from build123d import *

# Parameters (mm, degrees)
SKETCH2_R           = 1.75
SKETCH2_R_2         = 1.995
BOSS_EXTRUDE1_DEPTH = 4
SKETCH4_R           = 1.3
SKETCH4_R_2         = 2.4
CUT_EXTRUDE1_DEPTH  = 5


with BuildPart() as part:
    # Sketch2 → Boss-Extrude1 (new body)
    with BuildSketch(Plane.XY):
        with BuildLine():
            ThreePointArc((30.75, -4), (34.75, 0), (30.75, 4))
            Line((30.75, 4), (14.072558403, 4))
            ThreePointArc((14.072558403, 4), (14.06038767, 4.04257326), (14.048088143, 4.085109489))
            ThreePointArc((14.048088143, 4.085109489), (12.709169027, 4.272836063), (11.365584201, 4.122086336))
            ThreePointArc((11.365584201, 4.122086336), (11.169703548, 4.626642697), (10.951436862, 5.12192646))
            ThreePointArc((10.951436862, 5.12192646), (12.008090957, 5.965388247), (12.82210701, 7.044889767))
            ThreePointArc((12.82210701, 7.044889767), (12.669951657, 7.315), (12.51210701, 7.581825517))
            ThreePointArc((12.51210701, 7.581825517), (11.170223244, 7.416617696), (9.911436862, 6.9232593))
            ThreePointArc((9.911436862, 6.9232593), (9.591641884, 7.359925677), (9.252623584, 7.781841479))
            ThreePointArc((9.252623584, 7.781841479), (10.05496909, 8.870045207), (10.561852666, 10.123446462))
            ThreePointArc((10.561852666, 10.123446462), (10.344972209, 10.344972209), (10.123446462, 10.561852666))
            ThreePointArc((10.123446462, 10.561852666), (8.870045207, 10.05496909), (7.781841479, 9.252623584))
            ThreePointArc((7.781841479, 9.252623584), (7.359925677, 9.591641884), (6.9232593, 9.911436862))
            ThreePointArc((6.9232593, 9.911436862), (7.416617696, 11.170223244), (7.581825517, 12.51210701))
            ThreePointArc((7.581825517, 12.51210701), (7.315, 12.669951657), (7.044889767, 12.82210701))
            ThreePointArc((7.044889767, 12.82210701), (5.965388247, 12.008090957), (5.12192646, 10.951436862))
            ThreePointArc((5.12192646, 10.951436862), (4.626642697, 11.169703548), (4.122086336, 11.365584201))
            ThreePointArc((4.122086336, 11.365584201), (4.272836063, 12.709169027), (4.085109489, 14.048088143))
            ThreePointArc((4.085109489, 14.048088143), (3.78652263, 14.131494839), (3.486235477, 14.208555951))
            ThreePointArc((3.486235477, 14.208555951), (2.654199937, 13.14288127), (2.112960617, 11.903927815))
            ThreePointArc((2.112960617, 11.903927815), (1.578061664, 11.986568374), (1.04, 12.04518576))
            ThreePointArc((1.04, 12.04518576), (0.837867713, 13.382005944), (0.31, 14.626715284))
            ThreePointArc((0.31, 14.626715284), (0, 14.63), (-0.31, 14.626715284))
            ThreePointArc((-0.31, 14.626715284), (-0.837867713, 13.382005944), (-1.04, 12.04518576))
            ThreePointArc((-1.04, 12.04518576), (-1.578061664, 11.986568374), (-2.112960617, 11.903927815))
            ThreePointArc((-2.112960617, 11.903927815), (-2.654199937, 13.14288127), (-3.486235477, 14.208555951))
            ThreePointArc((-3.486235477, 14.208555951), (-3.78652263, 14.131494839), (-4.085109489, 14.048088143))
            ThreePointArc((-4.085109489, 14.048088143), (-4.272836063, 12.709169027), (-4.122086336, 11.365584201))
            ThreePointArc((-4.122086336, 11.365584201), (-4.626642697, 11.169703548), (-5.12192646, 10.951436862))
            ThreePointArc((-5.12192646, 10.951436862), (-5.965388247, 12.008090957), (-7.044889767, 12.82210701))
            ThreePointArc((-7.044889767, 12.82210701), (-7.315, 12.669951657), (-7.581825517, 12.51210701))
            ThreePointArc((-7.581825517, 12.51210701), (-7.416617696, 11.170223244), (-6.9232593, 9.911436862))
            ThreePointArc((-6.9232593, 9.911436862), (-7.359925677, 9.591641884), (-7.781841479, 9.252623584))
            ThreePointArc((-7.781841479, 9.252623584), (-8.870045207, 10.05496909), (-10.123446462, 10.561852666))
            ThreePointArc((-10.123446462, 10.561852666), (-10.344972209, 10.344972209), (-10.561852666, 10.123446462))
            ThreePointArc((-10.561852666, 10.123446462), (-10.05496909, 8.870045207), (-9.252623584, 7.781841479))
            ThreePointArc((-9.252623584, 7.781841479), (-9.591641884, 7.359925677), (-9.911436862, 6.9232593))
            ThreePointArc((-9.911436862, 6.9232593), (-11.170223244, 7.416617696), (-12.51210701, 7.581825517))
            ThreePointArc((-12.51210701, 7.581825517), (-12.669951657, 7.315), (-12.82210701, 7.044889767))
            ThreePointArc((-12.82210701, 7.044889767), (-12.008090957, 5.965388247), (-10.951436862, 5.12192646))
            ThreePointArc((-10.951436862, 5.12192646), (-11.169703548, 4.626642697), (-11.365584201, 4.122086336))
            ThreePointArc((-11.365584201, 4.122086336), (-12.709169027, 4.272836063), (-14.048088143, 4.085109489))
            ThreePointArc((-14.048088143, 4.085109489), (-14.131494839, 3.78652263), (-14.208555951, 3.486235477))
            ThreePointArc((-14.208555951, 3.486235477), (-13.14288127, 2.654199937), (-11.903927815, 2.112960617))
            ThreePointArc((-11.903927815, 2.112960617), (-11.986568374, 1.578061664), (-12.04518576, 1.04))
            ThreePointArc((-12.04518576, 1.04), (-13.382005944, 0.837867713), (-14.626715284, 0.31))
            ThreePointArc((-14.626715284, 0.31), (-14.63, 0), (-14.626715284, -0.31))
            ThreePointArc((-14.626715284, -0.31), (-13.382005944, -0.837867713), (-12.04518576, -1.04))
            ThreePointArc((-12.04518576, -1.04), (-11.986568374, -1.578061664), (-11.903927815, -2.112960617))
            ThreePointArc((-11.903927815, -2.112960617), (-13.14288127, -2.654199937), (-14.208555951, -3.486235477))
            ThreePointArc((-14.208555951, -3.486235477), (-14.131494839, -3.78652263), (-14.048088143, -4.085109489))
            ThreePointArc((-14.048088143, -4.085109489), (-12.709169027, -4.272836063), (-11.365584201, -4.122086336))
            ThreePointArc((-11.365584201, -4.122086336), (0.064808849, -12.089826294), (11.409123542, -4))
            Line((11.409123542, -4), (30.75, -4))
        make_face()
        Circle(SKETCH2_R, mode=Mode.SUBTRACT)
        with Locations((30.75, 0)):
            Circle(SKETCH2_R_2, mode=Mode.SUBTRACT)
    extrude(amount=BOSS_EXTRUDE1_DEPTH)

    # Sketch4 → Cut-Extrude1 (cut, through all)
    with BuildSketch(Plane.XY.offset(4)):
        with Locations((4.5, 0)):
            Circle(SKETCH4_R)
        with Locations((-4.5, 0)):
            Circle(SKETCH4_R)
        Circle(SKETCH4_R_2)
    extrude(amount=-CUT_EXTRUDE1_DEPTH, mode=Mode.SUBTRACT)


solid = part.part
Design review of the part built by this model. Coordinates are the model's own, in mm. A direction names the side the tool comes from. Round coordinates to 2 decimals unless told otherwise and drop trailing zeros. Write each loop counter-clockwise with the first axis right and the second up, starting at its lowest first coordinate (ties: lowest second). Pieces come first, ordered by that corner, then holes. Notation, with made-up numbers: M 46,15 L 71,15 A26 cw 71,51 Z; hole C 6,-28 d4. An arc over 180 degrees is marked long. One line per item, written item: value. Start each with the question number.
1. Take a section at B-B on x = 18.5. State the section outline as (y, z) points.
2. Clearance check with flat-ended pins moving along their axes: P1, Ø5.5, axis at x = 0, y = 0, coming from the -Z side; P2, Ø1.5, axis at x = 7, z = 0.5, coming from the -Y side; P3, Ø2, axis at x = 23, z = 2, coming from the -Y side; P4, Ø1.5, axis at y = 10, z = 2.5, coming from the +X side. State where each tip first meets the part, or that it passes through.
3. To check wall thickness, follow probe 1 along Y at (x, z) = (30.75, 2.2) (3 decimals); probe 2 along X at (y, z) = (-1.5, 1.85); probe 3 along Y at (x, z) = (0, 2.7). State the ranges of each line that lie inside material, in increasing order. Write a range as from..to.
4. Draft analysis for pull direction X (two halves, no side actions). For faces 4 (the face through (-8.853, 10.046, 1.972)), 5 (the face through (-11.986, 1.586, 1.972)), 6 (the face through (10.046, 8.853, 1.972)), state which applies: pulls with the +X half, pulls with the -X half, needs draft (parallel to the pull), parting line crosses it, or undercut.
5. For faces 1 (the face through (-10.064, 8.887, 1.972)), 2 (the face through (-12.69, 4.273, 1.972)), 3 (the face through (2.664, 13.159, 1.972)), list the 3-axis set-ups (+Z, -Z, +X, -X, +Y, -Y) from which the entire face can be reached by the end or side of a thin tool; tool diameter is ignored.
6. Take a section at A-A on z = 1.5. State how many separate pieces and enclosed holes the cut face has, then the cut area to 3 significant figures.
7. Take a section at C-C on y = -6.75. State the section outline as (x, z) points.
Computed:
1. outline: M -4,0 L 4,0 L 4,4 L -4,4 Z
2. P1: stops at z = 0
2. P2: stops at y = -10.35
2. P3: stops at y = -4
2. P4: stops at x = 10.56
3. probe 1: y = -4..-1.995, 1.995..4
3. probe 2: x = -12..-1.87, 1.87..29.43, 32.07..34.46
3. probe 3: y = -12.09..-2.4, 2.4..14.63
4. face 4: undercut
4. face 5: pulls with the -X half
4. face 6: pulls with the +X half
5. face 1: +Z, -Z, -X
5. face 2: +Z, -Z
5. face 3: +Z, -Z, +Y
6. separate pieces: 1
6. enclosed holes: 4
6. area: 643 mm²
7. outline: M -10.03,0 L 10.03,0 L 10.03,4 L -10.03,4 Z
